Could you check a few things on this model? Use its own coordinates, in mm. A direction names the side the tool comes from. Coordinates: 2 decimals unless noted, no trailing zeros. Order: outer loops, then holes, each group sorted by start corner. A loop starts at its lowest first (then second) coordinate and runs counter-clockwise, first axis right, second up. Notation, with made-up numbers: (54, 61.25) - (100, 61.25) arc R15 cw to (100, 89.25) - close; hole circle Ø3 at (20.5, 79). An arc over 180 degrees is marked (long way). Answer as a JSON object with one key per item and string values. Group by question number.
(1) Imagine slicing it at C-C, the plane x = -53.5. Write out the boundary of the cut face in (y, z) (3 decimals), and give its area (3 significant figures).
(2) Imagine slicing it at A-A, the plane z = 0. Write out the boundary of the cut face in (x, y) (3 decimals), and give its area (3 significant figures).
(3) Imagine slicing it at B-B, the plane y = -30.5. Write out the boundary of the cut face in (x, z) (3 decimals).
(4) Which directions (+Z, -Z, +X, -X, +Y, -Y) give clear straight access to the entire face, cutting with the end or side of a thin tool? Please do faces 1 (the flat face through (-136, -25, 0)), 2 (the flat face through (-93, -34, -9.525)), 3 (the cylindrical face through (9.523, -34.392, -0.209)), 4 (the flat face through (-1, -8, -51)).
(5) Imagine slicing it at D-D, the plane z = 42. Write out the boundary of the cut face in (x, y), and give its area (3 significant figures).
(6) Please list where these lines run through material, in increasing order: probe 1 along Z at (x, y) = (-43, -27) (3 decimals); probe 2 along Y at (x, z) = (36.5, 24); probe 3 along Y at (x, z) = (-56, -34.5).
(7) Will these pins go through, and if not, where does the flat tip stop? P1, Ø6, axis at x = -32.5, y = -7, coming from the -Z side; P2, Ø15, axis at x = -155, z = -0.5, coming from the +Y side; P3, Ø15, axis at x = -74.5, y = -34, coming from the -Z side (3 decimals).
from build123d import *

# Parameters (mm, degrees)
F0_R     = 50.8
F1_DEPTH = 8
F2_R     = 78
F2_R_2   = 50.8
F3_DEPTH = 17
F5_DEPTH = 19.05


with BuildPart() as f1:
    # F0 (on Front) → F1 (new body)
    with BuildSketch(Plane.XZ):
        Circle(F0_R)
    extrude(amount=F1_DEPTH)

    # F2 (on face) → F3 (join)
    with BuildSketch(Plane.XZ.offset(8)):
        Circle(F2_R)
        Circle(F2_R_2, mode=Mode.SUBTRACT)
        Circle(F2_R_2)
    extrude(amount=F3_DEPTH)

    # F4 (on face) → F5 (join)
    with BuildSketch(Plane.XZ.offset(25)):
        with BuildLine():
            ThreePointArc((-78, 0), (-77.853923, 4.771436), (-77.416241, 9.525))
            Line((-77.416241, 9.525), (-182.475, 9.525))
            ThreePointArc((-182.475, 9.525), (-192, 0), (-182.475, -9.525))
            Line((-182.475, -9.525), (-77.416241, -9.525))
            ThreePointArc((-77.416241, -9.525), (-77.853923, -4.771436), (-78, 0))
        make_face()
        with BuildLine():
            ThreePointArc((0, -9.525), (9.525, 0), (0, 9.525))
            Line((0, 9.525), (-77.416241, 9.525))
            ThreePointArc((-77.416241, 9.525), (-77.853923, 4.771436), (-78, 0))
            ThreePointArc((-78, 0), (-77.853923, -4.771436), (-77.416241, -9.525))
            Line((-77.416241, -9.525), (0, -9.525))
        make_face()
    extrude(amount=F5_DEPTH)


solid = f1.part
Result set:
{
 "1": {"outline": "(-44.05, -9.525) - (-25, -9.525) - (-25, -56.76) - (-8, -56.76) - (-8, 56.76) - (-25, 56.76) - (-25, 9.525) - (-44.05, 9.525) - close", "area": "2,290 mm^2"},
 "2": {"outline": "(-192, -44.05) - (9.525, -44.05) - (9.525, -25) - (78, -25) - (78, -8) - (50.8, -8) - (50.8, 0) - (-50.8, 0) - (-50.8, -8) - (-78, -8) - (-78, -25) - (-192, -25) - close", "area": "7,300 mm^2"},
 "3": {"outline": "(-182.475, -9.525) - (0, -9.525) arc R9.525 ccw to (0, 9.525) - (-182.475, 9.525) arc R9.525 ccw to start"},
 "4": {"face 1": "+Z, -Z, -X, +Y", "face 2": "-Z, +X, -X, -Y", "face 3": "+X, -Y", "face 4": "+Y"},
 "5": {"outline": "(-65.73, -25) - (65.73, -25) - (65.73, -8) - (28.58, -8) - (28.58, 0) - (-28.58, 0) - (-28.58, -8) - (-65.73, -8) - close", "area": "2,690 mm^2"},
 "6": {"probe 1": "z = -9.525 to 9.525", "probe 2": "y = -25 to 0", "probe 3": "y = -25 to -8"},
 "7": {"P1": "stops at z = -72.14", "P2": "stops at y = -25", "P3": "stops at z = -9.525"}
}
